from build123d import *

# Parameters (mm, degrees)
PAD_DEPTH       = 10
POCKET_DEPTH    = 9.5
SKETCH002_R     = 13.5
POCKET001_DEPTH = 1
SKETCH003_W     = 4.9
SKETCH003_H     = 10
PAD001_DEPTH    = 5
POCKET002_DEPTH = 10
SKETCH008_R     = 0.6
POCKET003_DEPTH = 2
SKETCH009_R     = 0.6
POCKET004_DEPTH = 2
FILLET_R        = 3.9
FILLET001_R     = 3.9
FILLET002_R     = 5
FILLET003_R     = 5
FILLET004_R     = 5
FILLET005_R     = 5
SKETCH010_W     = 3.45
SKETCH010_H     = 10
PAD002_DEPTH    = 6
POCKET005_DEPTH = 10
SKETCH012_R     = 0.6
POCKET006_DEPTH = 2
SKETCH013_R     = 0.6
POCKET007_DEPTH = 2
FILLET006_R     = 5.9
FILLET007_R     = 5.9


with BuildPart() as part:
    # Sketch → Pad (new body)
    with BuildSketch(Plane.XY):
        with BuildLine():
            Line((-21.862293, 15.5), (-21.862293, -15.5))
            Line((-21.862293, -15.5), (-15.125083, -17.4))
            ThreePointArc((-15.125083, -17.4), (0.226102, -23.053785), (15.463446, -17.1))
            Line((15.463446, -17.1), (22.461838, -16.95))
            Line((22.461838, 16.95), (22.461838, -16.95))
            Line((15.463446, 17.1), (22.461838, 16.95))
            ThreePointArc((15.463446, 17.1), (0.226102, 23.053785), (-15.125083, 17.4))
            Line((-21.862293, 15.5), (-15.125083, 17.4))
        make_face()
    extrude(amount=PAD_DEPTH)

    # Sketch001 → Pocket (cut)
    with BuildSketch(Plane.XY):
        with BuildLine():
            Line((-14.55, 16.55), (-20.805997, 15.2))
            Line((-20.805997, 15.2), (-20.805997, -15.2))
            Line((-20.805997, -15.2), (-14.55, -16.55))
            ThreePointArc((-14.55, -16.55), (0, -22.036447), (14.55, -16.55))
            Line((14.55, -16.55), (21.832857, -16.05))
            Line((21.832857, 16.05), (21.832857, -16.05))
            Line((14.55, 16.55), (21.832857, 16.05))
            ThreePointArc((14.55, 16.55), (0, 22.036447), (-14.55, 16.55))
        make_face()
    extrude(amount=POCKET_DEPTH, mode=Mode.SUBTRACT)

    # Sketch002 (on Face19 of Pocket) → Pocket001 (cut)
    with BuildSketch(Plane(origin=(0, 0, 9.5), x_dir=(1, 0, 0), z_dir=(0, 0, -1))):
        Circle(SKETCH002_R)
    extrude(amount=-POCKET001_DEPTH, mode=Mode.SUBTRACT)

    # Sketch003 (on Face6 of Pocket001) → Pad001 (join)
    with BuildSketch(Plane.YZ.offset(22.461838)):
        with Locations((-14.5, 5)):
            Rectangle(SKETCH003_W, SKETCH003_H)
        with Locations((14.5, 5)):
            Rectangle(SKETCH003_W, SKETCH003_H)
    extrude(amount=PAD001_DEPTH)

    # Sketch006 → Pocket002 (cut)
    with BuildSketch(Plane.XY.offset(10)):
        with BuildLine():
            ThreePointArc((22.461838, 16.95), (24.723382, 15.046575), (27.461838, 13.93371))
            Line((27.461838, 16.95), (27.461838, 13.93371))
            Line((27.461838, 16.95), (22.461838, 16.95))
        make_face()
        with BuildLine():
            ThreePointArc((27.461838, -13.93371), (24.723382, -15.046575), (22.461838, -16.95))
            Line((27.461838, -16.95), (22.461838, -16.95))
            Line((27.461838, -13.93371), (27.461838, -16.95))
        make_face()
    extrude(amount=-POCKET002_DEPTH, mode=Mode.SUBTRACT)

    # Sketch008 (on Face27 of Pocket002) → Pocket003 (cut)
    with BuildSketch(Plane(origin=(0, -12.05, 0), x_dir=(-1, 0, 0), z_dir=(0, 1, 0))):
        with Locations((-25.761838, 1.2)):
            Circle(SKETCH008_R)
    extrude(amount=-POCKET003_DEPTH, mode=Mode.SUBTRACT)

    # Sketch009 (on Face26 of Pocket003) → Pocket004 (cut)
    with BuildSketch(Plane.XZ.offset(-12.05)):
        with Locations((25.761838, 1.2)):
            Circle(SKETCH009_R)
    extrude(amount=-POCKET004_DEPTH, mode=Mode.SUBTRACT)

    # Fillet
    fillet_edges = [part.edges().sort_by_distance(p)[0] for p in [
        (27.461838, -12.991855, 10),
    ]]
    fillet(fillet_edges, radius=FILLET_R)

    # Fillet001
    fillet001_edges = [part.edges().sort_by_distance(p)[0] for p in [
        (27.461838, 12.991855, 10),
    ]]
    fillet(fillet001_edges, radius=FILLET001_R)

    # Fillet002
    fillet002_edges = [part.edges().sort_by_distance(p)[0] for p in [
        (15.463446, -17.1, 5),
    ]]
    fillet(fillet002_edges, radius=FILLET002_R)

    # Fillet003
    fillet003_edges = [part.edges().sort_by_distance(p)[0] for p in [
        (15.463446, 17.1, 5),
    ]]
    fillet(fillet003_edges, radius=FILLET003_R)

    # Fillet004
    fillet004_edges = [part.edges().sort_by_distance(p)[0] for p in [
        (-15.125083, -17.4, 5),
    ]]
    fillet(fillet004_edges, radius=FILLET004_R)

    # Fillet005
    fillet005_edges = [part.edges().sort_by_distance(p)[0] for p in [
        (-15.125083, 17.4, 5),
    ]]
    fillet(fillet005_edges, radius=FILLET005_R)

    # Sketch010 (on Face4 of Fillet005) → Pad002 (join)
    with BuildSketch(Plane(origin=(-21.862293, 0, 0), x_dir=(0, -1, 0), z_dir=(-1, 0, 0))):
        with Locations((-13.775, 5)):
            Rectangle(SKETCH010_W, SKETCH010_H)
        with Locations((13.775, 5)):
            Rectangle(SKETCH010_W, SKETCH010_H)
    extrude(amount=PAD002_DEPTH)

    # Sketch011 (on Face6 of Pad002) → Pocket005 (cut)
    with BuildSketch(Plane.XY.offset(10)):
        with BuildLine():
            ThreePointArc((-27.862293, 14.1), (-24.766364, 14.388874), (-21.862293, 15.5))
            Line((-21.862293, 15.5), (-27.862293, 15.5))
            Line((-27.862293, 15.5), (-27.862293, 14.1))
        make_face()
        with BuildLine():
            ThreePointArc((-21.862293, -15.5), (-24.766364, -14.388874), (-27.862293, -14.1))
            Line((-27.862293, -14.1), (-27.862293, -15.5))
            Line((-27.862293, -15.5), (-21.862293, -15.5))
        make_face()
    extrude(amount=-POCKET005_DEPTH, mode=Mode.SUBTRACT)

    # Sketch012 (on Face23 of Pocket005) → Pocket006 (cut)
    with BuildSketch(Plane(origin=(0, -12.05, 0), x_dir=(-1, 0, 0), z_dir=(0, 1, 0))):
        with Locations((26.162293, 1.2)):
            Circle(SKETCH012_R)
    extrude(amount=-POCKET006_DEPTH, mode=Mode.SUBTRACT)

    # Sketch013 (on Face21 of Pocket006) → Pocket007 (cut)
    with BuildSketch(Plane.XZ.offset(-12.05)):
        with Locations((-26.162293, 1.2)):
            Circle(SKETCH013_R)
    extrude(amount=-POCKET007_DEPTH, mode=Mode.SUBTRACT)

    # Fillet006
    fillet006_edges = [part.edges().sort_by_distance(p)[0] for p in [
        (-27.862293, 13.075, 10),
    ]]
    fillet(fillet006_edges, radius=FILLET006_R)

    # Fillet007
    fillet007_edges = [part.edges().sort_by_distance(p)[0] for p in [
        (-27.862293, -13.075, 10),
    ]]
    fillet(fillet007_edges, radius=FILLET007_R)


solid = part.part
Can you work these out from the model? Positions are in its coordinate system, mm. A direction names the side the tool comes from. Round coordinates to 2 decimals unless told otherwise and drop trailing zeros. Loops run counter-clockwise (first coordinate to the right, second up) from the corner with the lowest first, then second, coordinate; pieces in that order, holes last. Notation, with made-up numbers: (-27, 52) - (-5, 52) arc R26 ccw to (-5, 82) - close; hole circle Ø3 at (-23, 41). An arc over 180 degrees is marked (long way). Use CSV: the item, a comma, the result in double quotes. Start each with the question number.
1) If we section it at D-D on x = 18: Write out the boundary of the cut face in (y, z).
2) For faces 4 (the cylindrical face through (-15.23, -17.47, 5.07)), 5 (the flat face through (25, 12.05, 5)), 6 (the flat face through (-17.634, 15.884, 4.684)), 7 (the flat face through (26, 14.05, 1)), which set-ups out of +Z, -Z, +X, -X, +Y, -Y let a thin tool reach every point of the face, with its end or its side?
3) If we section it at A-A on x = 0: Write out the boundary of the cut face in (y, z), plus the area to 3 significant figures.
4) If we section it at B-B on y = 0: Write out the boundary of the cut face in (x, z).
5) Please list where these lines run through material, in increasing order: probe 1 along X at (y, z) = (-0.5, 4.5); probe 2 along Y at (x, z) = (-0.5, 6.75); probe 3 along Y at (x, z) = (0, 9.7). Write a range as [from, to].
6) We'd pull the mould along Z, two halves only. Please class faces 1 (the flat face through (-9, 11, 10)), 2 (the flat face through (-17.722, -15.866, 4.684)), 3 (the flat face through (26, -14.05, 1)): released by +Z, released by -Z, zero draft, split by the parting line, or undercut.
7) For pin 1 Ø0.7 at (x, z) = (-26.16, 1.2) entering from +Y; pin 2 Ø12 at (x, y) = (-5.5, -6) entering from -Z; pin 3 Ø1.1 at (x, z) = (25.76, 1.2) entering from -Y; pin 4 Ø1.5 at (x, y) = (7.5, 9.5) entering from -Z, each with a flat end and sliding along its axis, tell me the tip position at first contact or that it passes through.
Geometry results:
1,outline,"(-17.05, 0) - (-16.31, 0) - (-16.31, 9.5) - (16.31, 9.5) - (16.31, 0) - (17.05, 0) - (17.05, 10) - (-17.05, 10) - close"
2,face 4,"+Z, -Z, -X, -Y"
2,face 5,"+Z, -Z, +X"
2,face 6,"-Z"
2,face 7,"none"
3,outline,"(-23.05, 0) - (-22.04, 0) - (-22.04, 9.5) - (-13.5, 9.5) - (-13.5, 10) - (-23.05, 10) - close; (13.5, 9.5) - (22.04, 9.5) - (22.04, 0) - (23.05, 0) - (23.05, 10) - (13.5, 10) - close"
3,area,"28.9 mm2"
4,outline,"(-21.86, 0) - (-20.81, 0) - (-20.81, 9.5) - (-13.5, 9.5) - (-13.5, 10) - (-21.86, 10) - close; (13.5, 9.5) - (21.83, 9.5) - (21.83, 0) - (22.46, 0) - (22.46, 10) - (13.5, 10) - close"
5,probe 1,"x = [-21.86, -20.81], [21.83, 22.46]"
5,probe 2,"y = [-23.05, -22.03], [22.03, 23.05]"
5,probe 3,"y = [-23.05, -13.5], [13.5, 23.05]"
6,face 1,"released by +Z"
6,face 2,"zero draft"
6,face 3,"undercut"
7,pin 1,"stops at y = 14.2"
7,pin 2,"stops at z = 9.5"
7,pin 3,"stops at y = -14.77"
7,pin 4,"passes through"
